The listing builds one solid part. Answer for the finished solid, in the listing's coordinates (mm). Face numbers are marked on the shaded views. A direction names the side the tool comes from. Coordinates: 2 decimals unless noted, no trailing zeros. Loops run counter-clockwise (first coordinate to the right, second up) from the corner with the lowest first, then second, coordinate; pieces in that order, holes last. Notation, with made-up numbers: M 75,7.5 L 90,7.5 A32 cw 90,38.5 Z; hole C -20,5 d11. An arc over 180 degrees is marked long. Answer as CSV lines item,"result". Start each with the question number.
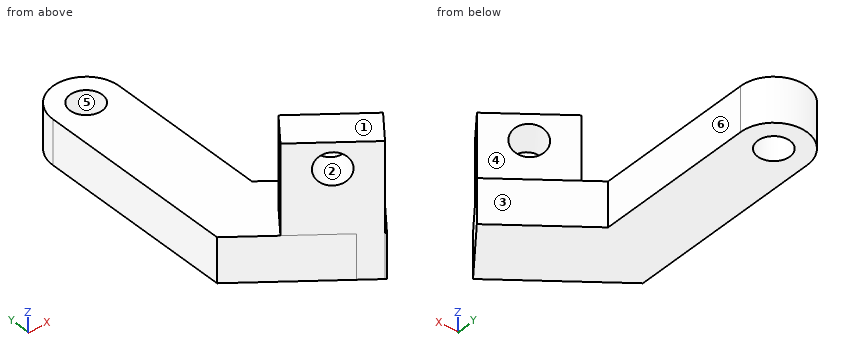
Autodesk Inventor part; units mm, degrees
ref_plane "YZ Plane" through (0, 0, 0) normal (1, 0, 0) x (0, 1, 0)
ref_plane "XZ Plane" through (0, 0, 0) normal (0, 1, 0) x (-1, 0, 0)
ref_plane "XY Plane" through (0, 0, 0) normal (0, 0, 1) x (1, 0, 0)
sketch "Szkic1" plane through (0, 0, 0) normal (0, 0, 1) x (1, 0, 0)
  circle A0 centre (26.2, 0.975) radius 1.45
  circle A1 centre (26.2, 0.975) radius 3
  line L0 (29.2, 0.975) -> (29.2, -8.7925)
  line L1 (23.2, -7.0757) -> (23.2, 0.975)
  line L2 (16.8275, -11.925) -> (-16.8275, 13.875) construction
  line L3 (23.2, -7.0757) -> (23.2, -16.8102)
  line L4 (23.2, -16.8102) -> (32.5797, -24.0007)
  line L5 (32.5797, -24.0007) -> (36.4465, -18.9567)
  line L6 (36.4465, -18.9567) -> (29.2, -13.4015)
  line L7 (29.2, -13.4015) -> (29.2, -8.7925)
  point P0 (0, 0)
  point P1 (29.2, -14.7925)
  point P2 (18.5681, -14.7925)
  point P3 (15.1107, -9.0757)
  point P4 (23.2, -9.0757)
  dimension "d5" = 6
  dimension "d12" = 2
  dimension "d13" = 6
extrude "Wyciągnięcie proste1" add sketch "Szkic1" along normal blind 4
sketch "Szkic4" plane through (0, 0, 4) normal (0, 0, 1) x (1, 0, 0)
  line L0 (34.4685, -21.3117) -> (28.6942, -16.8851)
  line L1 (16.8275, -11.925) -> (-16.8275, 13.875) construction
  line L2 (28.6942, -16.8851) -> (26.6967, -19.4907)
  line L3 (26.6967, -19.4907) -> (32.471, -23.9174)
  line L4 (32.471, -23.9174) -> (34.4685, -21.3117)
  line L5 (15.6301, -11.0071) -> (20.5681, -14.7925)
  line L6 (17.1107, -9.0757) -> (15.6301, -11.0071)
  point P0 (0, 0)
extrude "Wyciągnięcie proste2" add sketch "Szkic4" along normal blind 8 and the other way blind 4
sketch "Szkic6" plane through (23.2, -16.8102, 0) normal (-0.6084, -0.7936, 0) x (0.7936, -0.6084, 0)
  circle A0 centre (8.0439, 9.69) radius 1.45
  point P0 (-28.6395, 0)
  dimension "d21" = 2.9
extrude "Wyciągnięcie proste4" cut sketch "Szkic6" against normal blind 7
equation "\"d11\" = d7"
properties part number "mirror_arm_2"
Item 1: For a pull along Y with two mould halves and no side action, classify the marked faces 1, 2 and 3 as pulls with the +Y half, pulls with the -Y half, needs draft (parallel to the pull), parting line crosses it, or undercut.
Item 2: Section C-C on y = -12.75 is taken. Determine the outline of the cut face in (x, z), then the cut area to 3 significant figures.
Item 3: Section B-B on z = 4.5 is taken. Determine the outline of the cut face in (x, y).
Item 4: Section A-A on x = 26.2 is taken. Determine the outline of the cut face in (y, z) (3 decimals), then the cut area to 3 significant figures.
Item 5: For the marked faces 4, 5 and 6, determine the directions among +Z, -Z, +X, -X, +Y, -Y from which every point of the face is accessible in a straight line to the end or side of a thin tool.
Item 6: Consider line 1 (X direction, y = -7.5, z = 2); line 2 (Z direction, x = 27, y = -9); line 3 (Y direction, x = 26.2, z = 2.4) (3 decimals). Determine where each line is inside the solid, lowest interval first.
Item 7: Each of these flat-tipped pins is pushed along its axis until it touches: P1, Ø3, axis at x = 27.5, y = -6.5, coming from the +Z side; P2, Ø4, axis at y = -4.5, z = 2, coming from the +X side. Where does it stop, or does it pass through?
Results are:
1,face 1,"needs draft"
1,face 2,"undercut"
1,face 3,"pulls with the +Y half"
2,outline,"M 23.2,0 L 29.2,0 L 29.2,4 L 23.2,4 Z"
2,area,"24.0 mm²"
3,outline,"M 26.7,-19.49 L 32.47,-23.92 L 34.47,-21.31 L 28.69,-16.89 Z"
4,outline,"M -19.11,0 L -0.475,0 L -0.475,4 L -19.11,4 Z; M 2.425,0 L 3.975,0 L 3.975,4 L 2.425,4 Z"
4,area,"80.7 mm²"
5,face 4,"+Z, +X, +Y"
5,face 5,"+Z, -Z"
5,face 6,"+Z, -Z, +X, +Y"
6,line 1,"23.2 to 29.2"
6,line 2,"0 to 4"
6,line 3,"-19.11 to -0.475, 2.425 to 3.975"
7,P1,"z = 4"
7,P2,"x = 29.2"
